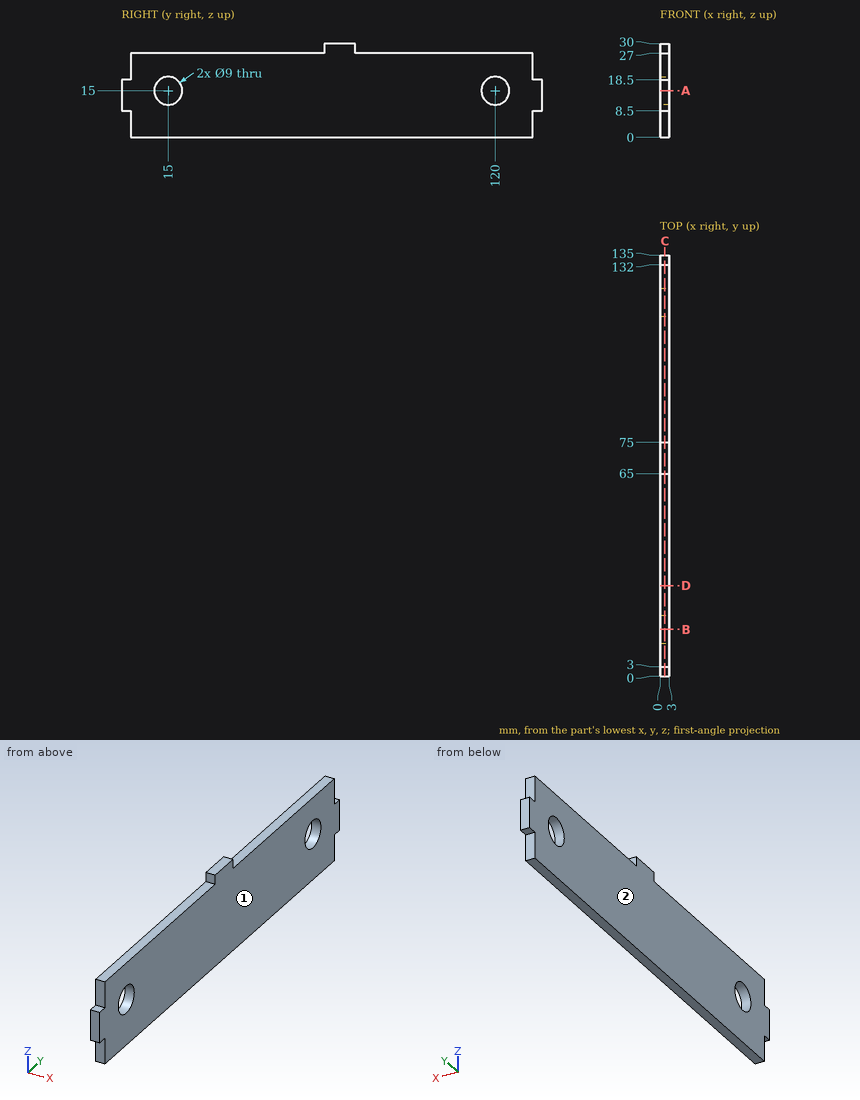
For this review, use the dimensioned drawing (mm, ordinates from the lowest corner) and the shaded views. Round coordinates to 2 decimals unless told otherwise and drop trailing zeros. Write each loop counter-clockwise with the first axis right and the second up, starting at its lowest first coordinate (ties: lowest second). Pieces come first, ordered by that corner, then holes. Notation, with made-up numbers: (-13, 51) - (21, 51) arc R20 ccw to (21, 87) - close; hole circle Ø5 at (89, -32.75). An arc over 180 degrees is marked (long way). Answer as a JSON object with one key per item and string values.
1. We need section C-C on x = 1.5. Give the boundary of the cut face in (y, z), then the cut area to 3 significant figures.
Response values:
{"outline": "(0, 8.5) - (3, 8.5) - (3, 0) - (132, 0) - (132, 8.5) - (135, 8.5) - (135, 18.5) - (132, 18.5) - (132, 27) - (75, 27) - (75, 30) - (65, 30) - (65, 27) - (3, 27) - (3, 18.5) - (0, 18.5) - close; hole circle Ø9 at (15, 15); hole circle Ø9 at (120, 15)", "area": "3,450 mm2"}
2. Draft analysis for pull direction X (two halves, no side actions). For the marked faces 1 and 2, state which applies: +X half, -X half, draft (parallel to the pull), parting line (faces both ways), or undercut.
Response values:
{"face 1": "+X half", "face 2": "-X half"}
3. To check wall thickness, follow line 1 along Y through (x, z) = (1.55, 15); line 2 along Y through (x, z) = (2.55, 17); line 3 along Z through (x, y) = (1.5, 117.5). State the ranges of each line that lie inside material, in increasing order.
Response values:
{"line 1": "y = 0 to 10.5, 19.5 to 115.5, 124.5 to 135", "line 2": "y = 0 to 10.97, 19.03 to 115.97, 124.03 to 135", "line 3": "z = 0 to 11.26, 18.74 to 27"}
4. We need section B-B on y = 15. Give the boundary of the cut face in (x, z), then the cut area to 3 significant figures.
Response values:
{"outline": "(0, 0) - (3, 0) - (3, 10.5) - (0, 10.5) - close; (0, 19.5) - (3, 19.5) - (3, 27) - (0, 27) - close", "area": "54.0 mm2"}
5. We need section A-A on z = 15. Give the boundary of the cut face in (x, y).
Response values:
{"outline": "(0, 0) - (3, 0) - (3, 10.5) - (0, 10.5) - close; (0, 19.5) - (3, 19.5) - (3, 115.5) - (0, 115.5) - close; (0, 124.5) - (3, 124.5) - (3, 135) - (0, 135) - close"}
6. For pin 1 Ø1.5 at (x, y) = (1.5, 26) entering from +Z; pin 2 Ø0.9 at (x, z) = (1, 28.5) entering from +Y; pin 3 Ø1.5 at (x, y) = (2, 2) entering from +Z, all flat-tipped, find the tip position at first contact; note any pin that passes through.
Response values:
{"pin 1": "stops at z = 27", "pin 2": "stops at y = 75", "pin 3": "stops at z = 18.5"}
7. We need section D-D on y = 29. Give the boundary of the cut face in (x, z), then the cut area to 3 significant figures.
Response values:
{"outline": "(0, 0) - (3, 0) - (3, 27) - (0, 27) - close", "area": "81.0 mm2"}
